Source: CAD feature listing. Evaluate the final solid. Frame: model axes, mm. A direction names the side the tool comes from. Give positions to 0.01 mm unless a question says otherwise; leave off trailing zeros. Loops run counter-clockwise (first coordinate to the right, second up) from the corner with the lowest first, then second, coordinate; pieces in that order, holes last. Notation, with made-up numbers: (2, 49) -> (20, 49) arc R23 cw to (20, 69) -> close; hole circle Ø6 at (4, -29.75). An arc over 180 degrees is marked (long way). Answer as a JSON object with one key per item and string values. Group by question number.
from build123d import *

# Parameters (mm, degrees)
SCHIZZO1_R                   = 17.5
ESTRUSIONE_ESTRUSIONE1_DEPTH = 31
RACCORDO1_R                  = 1
SCHIZZO2_R                   = 14.25
TAGLIO_ESTRUSIONE1_DEPTH     = 14
TAGLIO_ESTRUSIONE2_START     = -4.7
SCHIZZO5_R                   = 0.25
TAGLIO_ESTRUSIONE2_DEPTH     = 4.7
FORO_PER_VITE_M5_1_D         = 5.5


with BuildPart() as part:
    # Schizzo1 → Estrusione-Estrusione1 (new body)
    with BuildSketch(Plane.XY):
        Circle(SCHIZZO1_R)
    extrude(amount=ESTRUSIONE_ESTRUSIONE1_DEPTH)

    # Raccordo1
    raccordo1_edges = [part.edges().sort_by_distance(p)[0] for p in [
        (-17.5, 0, 31),
    ]]
    fillet(raccordo1_edges, radius=RACCORDO1_R)

    # Schizzo2 → Taglio-Estrusione1 (cut)
    with BuildSketch(Plane(origin=(0, 0, 0), x_dir=(-1, 0, 0), z_dir=(0, 0, -1))):
        Circle(SCHIZZO2_R)
    extrude(amount=-TAGLIO_ESTRUSIONE1_DEPTH, mode=Mode.SUBTRACT)

    # Schizzo3 → Taglia-Rivoluzione1 (revolve, cut)
    with BuildSketch(Plane(origin=(0, 0, 0), x_dir=(1, 0, 0), z_dir=(0, 1, 0)), mode=Mode.PRIVATE) as taglia_rivoluzione1_sk:
        Polygon((16, 0), (14.25, 0), (14.25, -6), align=None)
    revolve(taglia_rivoluzione1_sk.sketch.rotate(Axis((0, 0, 0), (0, 0, 1)), 180), axis=Axis((0, 0, 0), (0, 0, 1)), mode=Mode.SUBTRACT)

    # Schizzo4 → Taglia-Rivoluzione2 (revolve, cut)
    with BuildSketch(Plane(origin=(0, 0, 0), x_dir=(1, 0, 0), z_dir=(0, 1, 0)), mode=Mode.PRIVATE) as taglia_rivoluzione2_sk:
        Polygon((0.25, -18.7), (9.25, -14), (0.25, -14), align=None)
    revolve(taglia_rivoluzione2_sk.sketch.rotate(Axis((0, 0, 14), (0, 0, 1)), 180), axis=Axis((0, 0, 14), (0, 0, 1)), mode=Mode.SUBTRACT)

    # Schizzo5 → Taglio-Estrusione2 (cut)
    with BuildSketch(Plane(origin=(0, 0, 14), x_dir=(-1, 0, 0), z_dir=(0, 0, -1)).offset(TAGLIO_ESTRUSIONE2_START)):
        Circle(SCHIZZO5_R)
    extrude(amount=TAGLIO_ESTRUSIONE2_DEPTH, mode=Mode.SUBTRACT)

    # Foro per Vite M5-1 (through all)
    with Locations(Plane.XY.offset(31)):
        with Locations((0, 0)):
            Hole(FORO_PER_VITE_M5_1_D / 2)


solid = part.part
(1) Material intervals for line 1 (Y direction, x = 0, z = 20); line 2 (Y direction, x = 0, z = 7.5); line 3 (X direction, y = -12.5, z = 3), sorted ascending. Write a range as from..to.
(2) First-contact query: pin 1 (10 mm diameter, centred on x = -5.5, z = 22.5, fed in from +Y); pin 2 (10 mm diameter, centred on y = 9, z = 22, fed in from -X); pin 3 (2 mm diameter, centred on x = -10.5, z = 23, fed in from -Y); pin 4 (3.5 mm diameter, centred on x = 0, y = 0, fed in from -Z). Flat tips, straight axial feed; report the tip coordinate or a pass-through.
(3) Mould query, pull axis X, two halves, no side actions, for faces 1 (the face through (0.596, -2.685, 24.102)), 2 (the face through (-13.887, -10.648, 14.79)), 3 (the face through (7.7, -14.2, 0)). Classes: pulls with the +X half, pulls with the -X half, needs draft (parallel to the pull), parting line crosses it, or undercut.
(4) Access query for faces 4 (the face through (-13.163, -5.458, 9.944)), 5 (the face through (0, -3, 31)). Directions: +Z, -Z, +X, -X, +Y, -Y. A direction counts if a zero-diameter tool reaches every point of the face in a straight line with its end or side. Return the directions, or none.
(5) Section query C-C on z = 18. Return the cut outline in (x, y), plus the area to 3 significant figures.
(6) Section query A-A on x = 0. Return the cut outline in (y, z).
(7) Section query D-D on z = 3. Return the cut outline in (x, y) (3 decimals), plus the area to 3 significant figures.
Result:
{
 "1": {"line 1": "-17.5..-2.75, 2.75..17.5", "line 2": "-17.5..-14.25, 14.25..17.5", "line 3": "-12.25..-8.52, 8.52..12.25"},
 "2": {"pin 1": "y = 17.49", "pin 2": "x = -17.04", "pin 3": "y = -14.7", "pin 4": "through"},
 "3": {"face 1": "undercut", "face 2": "parting line crosses it", "face 3": "needs draft"},
 "4": {"face 4": "-Z", "face 5": "+Z, +X, -X, +Y, -Y"},
 "5": {"outline": "circle Ø35 at (0, 0); hole circle Ø5.5 at (0, 0)", "area": "938 mm²"},
 "6": {"outline": "(-17.5, 0) -> (-16, 0) -> (-14.25, 6) -> (-14.25, 14) -> (-9.25, 14) -> (-2.75, 17.39) -> (-2.75, 31) -> (-16.5, 31) arc R1 ccw to (-17.5, 30) -> close; (2.75, 17.39) -> (9.25, 14) -> (14.25, 14) -> (14.25, 6) -> (16, 0) -> (17.5, 0) -> (17.5, 30) arc R1 ccw to (16.5, 31) -> (2.75, 31) -> close"},
 "7": {"outline": "circle Ø35 at (0, 0); hole circle Ø30.25 at (0, 0)", "area": "243 mm²"}
}
